CAD build for the part. Positions are in the model's coordinates, mm. A direction names the side the tool comes from. Coordinates: 2 decimals unless noted, no trailing zeros. Loops run counter-clockwise (first coordinate to the right, second up) from the corner with the lowest first, then second, coordinate; pieces in that order, holes last.
1) Pin check, flat tips, straight feed: pin 1 Ø1.8 at (x, y) = (3, -0.5) entering from -Z; pin 2 Ø1.5 at (x, y) = (5.5, -3) entering from -Z; pin 3 Ø1.5 at (x, z) = (4, -35.5) entering from +Y; pin 4 Ø1.8 at (y, z) = (-1, 1) entering from +X. Stop position of each tip, or through.
2) Which spindle directions (+Z, -Z, +X, -X, +Y, -Y) get a long thin tool onto all of the face, cutting with end or side? Do faces 1 (the cylindrical face through (1, 0, -38)), 2 (the flat face through (3.648, 2.654, -1.504)). Say none if no direction does.
3) Wall check: line 1 along Z through (x, y) = (2.25, 0); line 2 along X through (y, z) = (0.5, -13); line 3 along Z through (x, y) = (4.5, 3.25). Give the ranges that are in metal, low to high.
4) Saw through at D-D, the plane z = -17. Write the cut outline in (x, y), and give its area (3 significant figures).
5) Saw through at A-A, the plane y = 0. Write the cut outline in (x, z).
6) Saw through at B-B, the plane x = 1.75. Write the cut outline in (y, z), and give its area (3 significant figures).
7) Saw through at C-C, the plane x = 5.5. Write the cut outline in (y, z).
8) Two-plate mould, pull along Z, no slides. Class faces 3 (the flat face through (7, 0.1, -3.3)), 4 (the cylindrical face through (4, 0, 5)), 5 (the flat face through (3.648, -2.629, -1.546)): +Z half, -Z half, draft (parallel to the pull), parting line (faces both ways), or undercut.
Autodesk Inventor part; units mm, degrees
ref_plane "YZ Plane" through (0, 0, 0) normal (1, 0, 0) x (0, 1, 0)
ref_plane "XZ Plane" through (0, 0, 0) normal (0, 1, 0) x (-1, 0, 0)
ref_plane "XY Plane" through (0, 0, 0) normal (0, 0, 1) x (1, 0, 0)
sketch "Boceto1" plane through (0, 0, 0) normal (1, 0, 0) x (0, 1, 0)
  arc A0 (5, 0) -> (-5, 0) centre (0, 0) ccw
  arc A1 (-5, -40) -> (5, -40) centre (0, -40) ccw
  line L0 (5, 0) -> (5, -40)
  line L1 (-5, -40) -> (-5, 0)
  circle A2 centre (0, -40) radius 2
  dimension "d1" = 10
  dimension "d2" = 10
  dimension "d3" = 40
  dimension "d4" = 4
extrude "Extrusión1" add sketch "Boceto1" along normal blind 3
sketch "Boceto2" plane through (3, 0, 0) normal (1, 0, 0) x (0, 0, -1)
  circle A0 centre (0, 0) radius 5
extrude "Extrusión2" add sketch "Boceto2" along normal blind 4
sketch "Boceto3" plane through (7, 0, 0) normal (1, 0, 0) x (0, 0, -1)
  line L0 (0, 3.5218) -> (3.05, 1.7609)
  line L1 (3.05, 1.7609) -> (3.05, -1.7609)
  line L2 (3.05, -1.7609) -> (0, -3.5218)
  line L3 (0, -3.5218) -> (-3.05, -1.7609)
  line L4 (-3.05, -1.7609) -> (-3.05, 1.7609)
  line L5 (-3.05, 1.7609) -> (0, 3.5218)
  point P0 (0, 0)
  point P1 (0, 0)
  point P2 (3.05, 0)
  dimension "d10" = 6.1
extrude "Extrusión3" cut sketch "Boceto3" against normal blind 6.8
properties part number "Transmision_Inf"
Data:
1. pin 1: stops at z = -45
1. pin 2: stops at z = -4.47
1. pin 3: passes through
1. pin 4: stops at x = 0.2
2. face 1: +X, -X
2. face 2: +X
3. line 1: z = -45 to -42, -38 to -3.05, 3.05 to 5
3. line 2: x = 0 to 3
3. line 3: z = -3.8 to -0.47, 0.47 to 3.8
4. outline: (0, -5) - (3, -5) - (3, 5) - (0, 5) - close
4. area: 30.0 mm2
5. outline: (0, -45) - (3, -45) - (3, -42) - (0, -42) - close; (0, -38) - (3, -38) - (3, -5) - (7, -5) - (7, -3.05) - (0.2, -3.05) - (0.2, 3.05) - (7, 3.05) - (7, 5) - (0, 5) - close
6. outline: (-5, -40) arc R5 ccw to (5, -40) - (5, 0) arc R5 ccw to (-5, 0) - close; hole (-3.52, 0) - (-1.76, -3.05) - (1.76, -3.05) - (3.52, 0) - (1.76, 3.05) - (-1.76, 3.05) - close; hole circle Ø4 at (0, -40)
6. area: 434 mm2
7. outline: circle Ø10 at (0, 0); hole (-3.52, 0) - (-1.76, -3.05) - (1.76, -3.05) - (3.52, 0) - (1.76, 3.05) - (-1.76, 3.05) - close
8. face 3: draft
8. face 4: parting line
8. face 5: undercut
